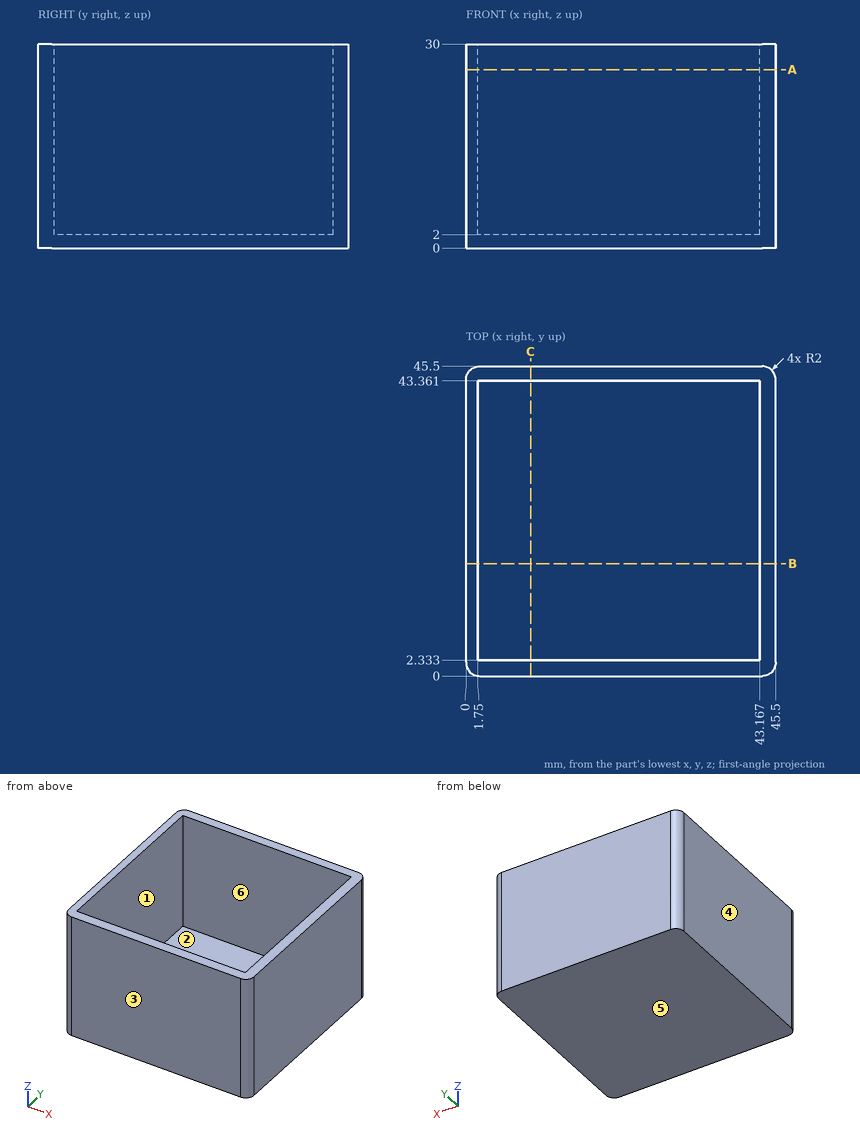
Answer from the drawing. Dimensions are ordinates in mm from the lowest x, y and z of the part. A direction names the side the tool comes from. Round coordinates to 2 decimals unless told otherwise and drop trailing zeros. Write each loop counter-clockwise with the first axis right and the second up, starting at its lowest first coordinate (ties: lowest second). Pieces come first, ordered by that corner, then holes. Notation, with made-up numbers: (36.25, 23.5) - (64.25, 23.5) arc R10 ccw to (64.25, 40.5) - close; hole circle Ø1 at (57, 69.25). An arc over 180 degrees is marked (long way). One line per item, written item: value.
Q1. Find section B-B (y = 16.5). Determine the outline of the cut face in (x, z).
The answers:
outline: (0, 0) - (45.5, 0) - (45.5, 30) - (43.17, 30) - (43.17, 2) - (1.75, 2) - (1.75, 30) - (0, 30) - close
Q2. Find section C-C (x = 9.5). Determine the outline of the cut face in (y, z).
The answers:
outline: (0, 0) - (45.5, 0) - (45.5, 30) - (43.36, 30) - (43.36, 2) - (2.33, 2) - (2.33, 30) - (0, 30) - close
Q3. Straight lines are drawn through the part: line 1 (X direction, y = 40, z = 13.25); line 2 (Y direction, x = 42, z = 16); line 3 (Z direction, x = 23.5, y = 32.5). For each, find the intervals that lie inside material, in ascending order. Write a range as from..to.
The answers:
line 1: x = 0..1.75, 43.17..45.5
line 2: y = 0..2.33, 43.36..45.5
line 3: z = 0..2
Q4. For a pull along X with two mould halves and no side action, classify the marked faces 1, 2, 3 and 4 as pulls with the +X half, pulls with the -X half, needs draft (parallel to the pull), parting line crosses it, or undercut.
The answers:
face 1: undercut
face 2: undercut
face 3: needs draft
face 4: pulls with the -X half
Q5. Which of the six approach directions +Z, -Z, +X, -X, +Y, -Y give full straight-line access (tool end or side, diameter ignored) to the marked faces 5 and 6?
The answers:
face 5: -Z, +X, -X, +Y, -Y
face 6: +Z
Q6. Find section A-A (z = 26.25). Determine the outline of the cut face in (x, y).
The answers:
outline: (0, 2) arc R2 ccw to (2, 0) - (43.5, 0) arc R2 ccw to (45.5, 2) - (45.5, 43.5) arc R2 ccw to (43.5, 45.5) - (2, 45.5) arc R2 ccw to (0, 43.5) - close; hole (1.75, 2.33) - (43.17, 2.33) - (43.17, 43.36) - (1.75, 43.36) - close
Q7. This flat-tipped pin is pushed along its axis until it touches: P1, Ø10, axis at x = 12.5, y = 33, coming from the +Z side. Where does it stop, or does it pass through?
The answers:
P1: stops at z = 2
